Geometry check sheet. Reference: the model listing, model coordinates, mm. A direction names the side the tool comes from. Round coordinates to 2 decimals unless told otherwise and drop trailing zeros. Loops run counter-clockwise (first coordinate to the right, second up) from the corner with the lowest first, then second, coordinate; pieces in that order, holes last. Notation, with made-up numbers: M 83.25,57.25 L 109.25,57.25 A33 ccw 109.25,94.25 Z; hole C -26.75,84 d7. An arc over 180 degrees is marked long. Use one line per item in the form item = value. Start each with the question number.
1. Cross-section at C-C (x = 21.5). Record the boundary of the cut face in (y, z).
2. Set-up check for faces 1 (the cylindrical face through (25.016, 11.674, 35.098)), 2 (the flat face through (-36, 12, 37)), 3 (the flat face through (30, 11, 52)): record each of +Z, -Z, +X, -X, +Y, -Y from which the full face is reachable in a straight line by a thin tool's end or side.
3. Draft check along Y on faces 4 (the cylindrical face through (-25.109, 11.874, 35.098)), 5 (the cylindrical face through (31.908, 0.601, -0.07)), 6 (the flat face through (-30, 11, 52)), 7 (the cylindrical face through (-28.092, 0.601, -0.07)). Enter one of: pulls with the +Y half, pulls with the -Y half, needs draft (parallel to the pull), parting line crosses it, or undercut.
4. Cross-section at B-B (y = 14.75). Record the boundary of the cut face in (x, z).
5. Material ranges on line 1 (Y direction, x = 30, z = 2.5); line 2 (Z direction, x = 28, y = 10.5); line 3 (X direction, y = 11.75, z = 59.5), recorded low to high.
6. Go/stop test with flat-tipped pins: pin 1 (3 mm diameter, centred on x = -3, z = 0, fed in from +Y); pin 2 (9 mm diameter, centred on x = 30.5, z = 64.5, fed in from -Y); pin 3 (2 mm diameter, centred on x = 22.5, z = 27, fed in from -Y); pin 4 (6 mm diameter, centred on x = 11, y = -1.5, fed in from +Z). Record where each tip stops, or that it passes through.
```python
from build123d import *

# Parameters (mm, degrees)
SKETCH1_R           = 2
BOSS_EXTRUDE1_DEPTH = 5
SKETCH1_3_W         = 10
SKETCH1_3_H         = 5
BOSS_EXTRUDE2_DEPTH = 100
FILLET1_R           = 10


with BuildPart() as part:
    # Sketch1 → Boss-Extrude1 (new, symmetric)
    with BuildSketch(Plane.XY):
        with BuildLine():
            ThreePointArc((-36, 0), (-34.242640687, -4.242640687), (-30, -6))
            Line((-30, -6), (30, -6))
            ThreePointArc((30, -6), (34.242640687, -4.242640687), (36, 0))
            Line((36, 0), (36, 16))
            Line((36, 16), (26, 16))
            Line((26, 16), (26, 6))
            Line((26, 6), (-26, 6))
            Line((-26, 6), (-26, 16))
            Line((-26, 16), (-36, 16))
            Line((-36, 16), (-36, 0))
        make_face()
        with Locations((-30, 0)):
            Circle(SKETCH1_R, mode=Mode.SUBTRACT)
        with Locations((30, 0)):
            Circle(SKETCH1_R, mode=Mode.SUBTRACT)
    extrude(amount=BOSS_EXTRUDE1_DEPTH, both=True)

    # Sketch1<3> → Boss-Extrude2 (add)
    with BuildSketch(Plane.XY):
        with Locations((-31, 13.5)):
            Rectangle(SKETCH1_3_W, SKETCH1_3_H)
        with Locations((31, 13.5)):
            Rectangle(SKETCH1_3_W, SKETCH1_3_H)
    extrude(amount=BOSS_EXTRUDE2_DEPTH)

    # Fillet1
    fillet1_edges = [part.edges().sort_by_distance(p)[0] for p in [
        (26, 6, 0),
        (-26, 6, 0),
    ]]
    fillet(fillet1_edges, radius=FILLET1_R - 0.0001)  # a hair under: the kernel refuses the full size


solid = part.part
```
Reported:
q1.outline = M -6,-5 L 7.65,-5 L 7.65,5 L -6,5 Z
q2.face_1 = +Z, -Z, +Y
q2.face_2 = +Z, -Z, -X, +Y, -Y
q2.face_3 = +Z, +X, -X, -Y
q3.face_4 = pulls with the +Y half
q3.face_5 = undercut
q3.face_6 = pulls with the -Y half
q3.face_7 = undercut
q4.outline = M -36,-5 L -25.92,-5 L -25.92,100 L -36,100 Z; M 25.92,-5 L 36,-5 L 36,100 L 25.92,100 Z
q5.line_1 = -6 to -2, 2 to 16
q5.line_2 = -5 to 5
q5.line_3 = -36 to -25.05, 25.05 to 36
q6.pin_1 = 6
q6.pin_2 = 11
q6.pin_3 = through
q6.pin_4 = 5
